The listing builds one solid part. Answer for the finished solid, in the listing's coordinates (mm). A direction names the side the tool comes from. Round coordinates to 2 decimals unless told otherwise and drop trailing zeros. Order: outer loops, then holes, each group sorted by start corner. A loop starts at its lowest first (then second) coordinate and runs counter-clockwise, first axis right, second up. Notation, with made-up numbers: M 52.25,86 L 95.25,86 A27 cw 95.25,110 Z; hole C 51.25,43.5 d7. An arc over 180 degrees is marked long. Write item = value, one per line. Start each with the question number.
(1) A cutting plane is placed at C-C, the plane x = 0. Determine the outline of the cut face in (y, z).
(2) Which of the six approach directions +Z, -Z, +X, -X, +Y, -Y give full straight-line access (tool end or side, diameter ignored) to faces 1 (the face through (8, 8, 0.6)), 2 (the face through (1.5, 8, -9)), 3 (the face through (0, 20, 0)), 4 (the face through (-1.5, 8, -9))?
(3) Straight lines are drawn through the part: probe 1 along X at (y, z) = (10.5, -0.9); probe 2 along X at (y, z) = (28, -0.9); probe 3 along Z at (x, y) = (0, 11.5). For each, find the intervals that lie inside material, in ascending order. Write a range as from..to.
(4) A cutting plane is placed at D-D, the plane x = -12.25. Determine the outline of the cut face in (y, z).
(5) A cutting plane is placed at A-A, the plane y = 9. Determine the outline of the cut face in (x, z).
(6) Each of these flat-tipped pins is pushed along its axis until it touches: pin 1 (12 mm diameter, centred on x = 9.5, y = 30.5, fed in from -Z); pin 2 (3.5 mm diameter, centred on x = -0.5, z = 7, fed in from +Y); pin 3 (10 mm diameter, centred on x = -3.5, z = 1, fed in from -Y); pin 4 (4 mm diameter, centred on x = 8.5, y = 5, fed in from -Z). Where does it stop, or does it pass through?
(7) A cutting plane is placed at B-B, the plane z = -0.9. Determine the outline of the cut face in (x, y), and give its area (3 significant figures).
(8) For a pull along X with two mould halves and no side action, classify faces 5 (the face through (15, 8, -1)), 6 (the face through (-8, 8, -2.4)), 7 (the face through (0, 19.7, -2.4)), 8 (the face through (-1.5, 8, 8)) as released by +X, released by -X, zero draft, split by the parting line, or undercut.
from build123d import *

# Parameters (mm, degrees)
BOSS_EXTRUDE1_DEPTH     = 17
BOSS_EXTRUDE2_START     = 17
BOSS_EXTRUDE2_OUTLINE_R = 2.5
BOSS_EXTRUDE2_DEPTH     = 23


# Read off the part's stored shape, not the designer's step: Boss-Extrude2
with BuildPart() as part:
    # Sketch1 → Boss-Extrude1 (new body)
    with BuildSketch(Plane(origin=(0, 0, 0), x_dir=(1, 0, 0), z_dir=(0, 1, 0))):
        with BuildLine():
            Line((-1.5, -1.1), (-1.5, -14.1))
            Line((-1.5, -14.1), (1.5, -14.1))
            Line((1.5, -14.1), (1.5, -1.1))
            ThreePointArc((1.5, -1.1), (1.767766953, -0.867766953), (2, -0.6))
            Line((2, -0.6), (15, -0.6))
            Line((15, -0.6), (15, 2.4))
            Line((15, 2.4), (2, 2.4))
            ThreePointArc((2, 2.4), (1.767766953, 2.667766953), (1.5, 2.9))
            Line((1.5, 2.9), (1.5, 15.9))
            Line((1.5, 15.9), (-1.5, 15.9))
            Line((-1.5, 15.9), (-1.5, 2.9))
            ThreePointArc((-1.5, 2.9), (-1.767766953, 2.667766953), (-2, 2.4))
            Line((-2, 2.4), (-15, 2.4))
            Line((-15, 2.4), (-15, -0.6))
            Line((-15, -0.6), (-2, -0.6))
            ThreePointArc((-2, -0.6), (-1.767766953, -0.867766953), (-1.5, -1.1))
        make_face()
        with BuildLine():
            ThreePointArc((-1.2, 0), (0, 2.4), (1.2, 0))
            Line((1.2, 0), (-1.2, 0))
        make_face(mode=Mode.SUBTRACT)
    extrude(amount=BOSS_EXTRUDE1_DEPTH)

    # Boss-Extrude2 outline → Boss-Extrude2 (add)
    with BuildSketch(Plane(origin=(0, 0, 0), x_dir=(1, 0, 0), z_dir=(0, 1, 0)).offset(BOSS_EXTRUDE2_START)):
        with Locations((0, 0.9)):
            Circle(BOSS_EXTRUDE2_OUTLINE_R)
        with BuildLine():
            Line((1.2, 0), (-1.2, 0))
            ThreePointArc((-1.2, 0), (0, 2.4), (1.2, 0))
        make_face(mode=Mode.SUBTRACT)
    extrude(amount=BOSS_EXTRUDE2_DEPTH)


solid = part.part
Reported:
q1.outline = M 0,-15.9 L 17,-15.9 L 17,-3.4 L 40,-3.4 L 40,-2.4 L 0,-2.4 Z; M 0,0 L 40,0 L 40,1.6 L 17,1.6 L 17,14.1 L 0,14.1 Z
q2.face_1 = +Z, +X, +Y, -Y
q2.face_2 = -Z, +X, +Y, -Y
q2.face_3 = +Y, -Y
q2.face_4 = -Z, -X, +Y, -Y
q3.probe_1 = -15..-1.5, 1.5..15
q3.probe_2 = -2.5..-1.5, 1.5..2.5
q3.probe_3 = -15.9..-2.4, 0..14.1
q4.outline = M 0,-2.4 L 17,-2.4 L 17,0.6 L 0,0.6 Z
q5.outline = M -15,-2.4 L -2,-2.4 A2.5 ccw -1.5,-2.9 L -1.5,-15.9 L 1.5,-15.9 L 1.5,-2.9 A2.5 ccw 2,-2.4 L 15,-2.4 L 15,0.6 L 2,0.6 A2.5 ccw 1.5,1.1 L 1.5,14.1 L -1.5,14.1 L -1.5,1.1 A2.5 ccw -2,0.6 L -15,0.6 Z; hole M -1.2,0 A1.5 ccw long 1.2,0 Z
q6.pin_1 = through
q6.pin_2 = 17
q6.pin_3 = 0
q6.pin_4 = -2.4
q7.outline = M -15,0 L -1.5,0 L -1.5,40 L -2.5,40 L -2.5,17 L -15,17 Z; M 1.5,0 L 15,0 L 15,17 L 2.5,17 L 2.5,40 L 1.5,40 Z
q7.area = 505 mm²
q8.face_5 = released by +X
q8.face_6 = zero draft
q8.face_7 = undercut
q8.face_8 = released by -X
